Read the model definition and answer for the solid it produces. Units are mm, in the model's axes. A direction names the side the tool comes from. Give positions to 0.01 mm unless a question says otherwise; leave off trailing zeros. Order: outer loops, then holes, each group sorted by start corner. A loop starts at its lowest first (then second) coordinate and runs counter-clockwise, first axis right, second up. Notation, with made-up numbers: (-12, 65.25) - (1, 65.25) arc R25 cw to (1, 103.25) - close; hole circle Ø4 at (43, 22.25). An arc over 180 degrees is marked (long way). Use a Markdown table: item, result. Add a question column.
1. Which of the six approach directions +Z, -Z, +X, -X, +Y, -Y give full straight-line access (tool end or side, diameter ignored) to faces 4 (the flat face through (15.875, -11.8, -4)), 5 (the cylindrical face through (19.14, -25.324, -9.842)), 6 (the cylindrical face through (-26.73, -18.11, 0.91))?
2. A cutting plane is placed at A-A on y = 30. Determine the outline of the cut face in (x, z).
3. A cutting plane is placed at D-D on x = 27. Determine the outline of the cut face in (y, z) (3 decimals).
4. A cutting plane is placed at C-C on x = 7. Determine the outline of the cut face in (y, z), and give its area (3 significant figures).
5. A cutting plane is placed at B-B on z = 0. State how many separate pieces and enclosed holes the cut face has, and give its area (3 significant figures).
6. Consider L1, parallel to X at y = -35, z = 10.5 (3 decimals); L2, parallel to Y at x = 0, z = -8.5 (3 decimals); L3, parallel to Y at x = 1.5, z = 9. Determine where each line is inside the solid, lowest interval first.
7. Flat-ended cylindrical pins translate along their axes: P1, Ø10, axis at x = -10.5, z = -10.5, coming from the -Y side; P2, Ø1.5, axis at x = 19, y = 29, coming from the +Z side; P3, Ø10, axis at x = -14, y = 36, coming from the +Z side. Find the tip coordinate at first contact, or state that the pin passes through.
8. For a pull along Y with two mould halves and no side action, classify faces 1 (the flat face through (-0.445, 14.266, 14.964)), 2 (the flat face through (-21.844, -22.4, 4.4)), 3 (the flat face through (-15.875, -11, 0)) as released by +Y, released by -Y, zero draft, split by the parting line, or undercut.
```python
from build123d import *

# Parameters (mm, degrees)
SKETCH1_R               = 9.525
BOSS_EXTRUDE1_DEPTH     = 19.05
SKETCH2_OUTSIDE_W       = 63.24
SKETCH2_OUTSIDE_H       = 114.04
CUT_EXTRUDE1_DEPTH      = 32.75
CUT_EXTRUDE1_DEPTH_BACK = 32.75


with BuildPart() as part:
    # Sketch1 → Boss-Extrude1 (new body, symmetric)
    with BuildSketch(Plane.XY):
        with BuildLine():
            Line((17.721167904, 35.565186559), (31.75, 0))
            Line((31.75, 0), (31.75, -41.275))
            Line((31.75, -41.275), (15.875, -41.275))
            Line((15.875, -41.275), (15.875, 0))
            Line((15.875, 0), (-15.875, 0))
            Line((-15.875, 0), (-15.875, -41.275))
            Line((-15.875, -41.275), (-31.75, -41.275))
            Line((-31.75, -41.275), (-31.75, 0))
            Line((-31.75, 0), (-17.721167904, 35.565186559))
            ThreePointArc((-17.721167904, 35.565186559), (0, 47.625), (17.721167904, 35.565186559))
        make_face()
        with Locations((0, 28.575)):
            Circle(SKETCH1_R, mode=Mode.SUBTRACT)
    extrude(amount=BOSS_EXTRUDE1_DEPTH, both=True)

    # Sketch2 outside → Cut-Extrude1 (cut, two sides)
    with BuildSketch(Plane(origin=(0, 0, 0), x_dir=(0, 0, -1), z_dir=(1, 0, 0))) as cut_extrude1_sk:
        with Locations((0, 3.175)):
            Rectangle(SKETCH2_OUTSIDE_W, SKETCH2_OUTSIDE_H)
        with BuildLine():
            Line((18.924303972, -20.040230177), (11.1125, 47.625))
            Line((11.1125, 47.625), (-11.1125, 47.625))
            Line((-11.1125, 47.625), (-18.924303972, -20.040230177))
            ThreePointArc((-18.924303972, -20.040230177), (0, -41.275), (18.924303972, -20.040230177))
        make_face(mode=Mode.SUBTRACT)
    extrude(amount=CUT_EXTRUDE1_DEPTH, mode=Mode.SUBTRACT)
    extrude(cut_extrude1_sk.sketch, amount=-CUT_EXTRUDE1_DEPTH_BACK, mode=Mode.SUBTRACT)

    # Sketch6 → CBORE for 5/16 Hex Head Bolt2 (revolve, cut)
    with BuildSketch(Plane(origin=(-15.875, -22.225, 0), x_dir=(0, 0, -1), z_dir=(0, 1, 0))):
        Polygon((0, 0), (0, 15.875), (4.2164, 15.875), (4.2164, 5.969), (10.31875, 5.969), (10.31875, 0.635), (10.95375, 0), align=None)
    cbore_for_5_16_hex_head_bolt2 = revolve(axis=Axis((-9.525, -22.225, 0), (-1, 0, 0)), mode=Mode.SUBTRACT)

    # Mirror1: CBORE for 5/16 Hex Head Bolt2 across plane
    add(cbore_for_5_16_hex_head_bolt2.mirror(Plane(origin=(0, 0, 0), x_dir=(0, 0, 1), z_dir=(1, 0, 0))), mode=Mode.SUBTRACT)


solid = part.part
```
Output values:
| question | item | result |
|---|---|---|
| 1 | face 4 | +Z, -Z, -Y |
| 1 | face 5 | none |
| 1 | face 6 | +X, -X |
| 2 | outline | (-19.92, -13.15) - (-9.42, -13.15) - (-9.42, 13.15) - (-19.92, 13.15) - close; (9.42, -13.15) - (19.92, -13.15) - (19.92, 13.15) - (9.42, 13.15) - close |
| 3 | outline | (-20.04, -18.924) - (12.042, -15.22) - (12.042, 15.22) - (-20.04, 18.924) arc R19.05 ccw (long way) to start; hole circle Ø8.433 at (-22.225, 0) |
| 4 | outline | (0, -16.61) - (22.12, -14.06) - (22.12, 14.06) - (0, 16.61) - close; (35.03, -12.57) - (46.29, -11.27) - (46.29, 11.27) - (35.03, 12.57) - close |
| 4 | area | 947 mm² |
| 5 | separate pieces | 3 |
| 5 | enclosed holes | 1 |
| 5 | area | 2,680 mm² |
| 6 | L1 | -31.75 to -15.875, 15.875 to 31.75 |
| 6 | L2 | 0 to 19.05, 38.1 to 47.625 |
| 6 | L3 | 0 to 19.17, 37.98 to 47.57 |
| 7 | P1 | y = 0 |
| 7 | P2 | z = 13.35 |
| 7 | P3 | z = 13.03 |
| 8 | face 1 | released by +Y |
| 8 | face 2 | undercut |
| 8 | face 3 | zero draft |
